Geometry check sheet. Reference: the model listing, model coordinates, mm. Face numbers are marked on the shaded views. A direction names the side the tool comes from. Give positions to 0.01 mm unless a question says otherwise; leave off trailing zeros. Order: outer loops, then holes, each group sorted by start corner. A loop starts at its lowest first (then second) coordinate and runs counter-clockwise, first axis right, second up.
from build123d import *

# Parameters (mm, degrees)
PAD_DEPTH       = 21
POCKET_DEPTH    = 5
POCKET001_DEPTH = 5
POCKET002_DEPTH = 10
SKETCH004_W     = 2.373045
SKETCH004_H     = 7.119136
POCKET003_DEPTH = 10
POCKET004_DEPTH = 10
POCKET005_DEPTH = 10
POCKET006_DEPTH = 2


with BuildPart() as part:
    # Sketch → Pad (new body)
    with BuildSketch(Plane.XY):
        Polygon((-10.032319, 15.304274), (9.936683, 15.304274), (19.912732, -0.173444), (9.919492, -15.052223), (9.919492, -25.320239), (-9.903072, -25.320239), (-9.903072, -15.596819), (-19.889567, -0.189549), align=None)
    extrude(amount=PAD_DEPTH)

    # Sketch001 (on Face10 of Pad) → Pocket (cut)
    with BuildSketch(Plane.XY.offset(21)):
        Polygon((-5.628046, 8.046473), (-9.278885, 3.056992), (-2.58568, 2.691908), align=None)
    extrude(amount=-POCKET_DEPTH, mode=Mode.SUBTRACT)

    # Sketch002 (on Face5 of Pocket) → Pocket001 (cut)
    with BuildSketch(Plane.XY.offset(21)):
        Polygon((6.8832, 8.120049), (3.658293, 3.373958), (10.594886, 3.069721), align=None)
    extrude(amount=-POCKET001_DEPTH, mode=Mode.SUBTRACT)

    # Sketch003 (on Face5 of Pocket001) → Pocket002 (cut)
    with BuildSketch(Plane.XY.offset(21)):
        Polygon((-7.814318, -23.860096), (-5.938107, -23.860096), (-5.938107, -16.355255), (-7.814318, -16.27368), align=None)
    extrude(amount=-POCKET002_DEPTH, mode=Mode.SUBTRACT)

    # Sketch004 (on Face5 of Pocket002) → Pocket003 (cut)
    with BuildSketch(Plane.XY.offset(21)):
        with Locations((-2.952688, -20.020277)):
            Rectangle(SKETCH004_W, SKETCH004_H)
    extrude(amount=-POCKET003_DEPTH, mode=Mode.SUBTRACT)

    # Sketch005 (on Face5 of Pocket003) → Pocket004 (cut)
    with BuildSketch(Plane.XY.offset(21)):
        Polygon((1.397894, -16.88661), (1.397894, -23.518969), (3.588397, -23.518969), (3.588397, -17.129999), align=None)
    extrude(amount=-POCKET004_DEPTH, mode=Mode.SUBTRACT)

    # Sketch006 (on Face5 of Pocket004) → Pocket005 (cut)
    with BuildSketch(Plane.XY.offset(21)):
        Polygon((5.109581, -16.88661), (5.474663, -23.701509), (7.847709, -23.823204), (7.847709, -16.460678), (5.474663, -16.704067), align=None)
    extrude(amount=-POCKET005_DEPTH, mode=Mode.SUBTRACT)

    # Sketch007 (on Face5 of Pocket005) → Pocket006 (cut)
    with BuildSketch(Plane.XY.offset(21)):
        Polygon((0, -2.312892), (-2.612413, -6.846357), (3.296795, -6.937919), align=None)
    extrude(amount=-POCKET006_DEPTH, mode=Mode.SUBTRACT)


solid = part.part
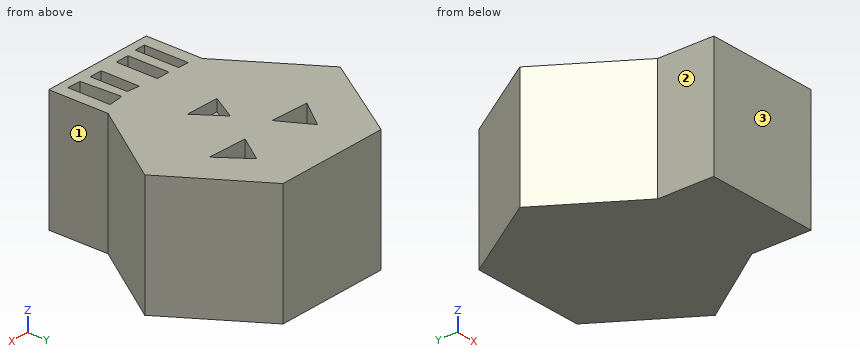
Item 1: Sectioned sample at C-C (y = 6.5). Enter the section's corners in (x, z), and give its area (3 significant figures).
Reported:
outline: (-15.63, 0) - (15.61, 0) - (15.61, 21) - (8.07, 21) - (8.07, 16) - (5.78, 16) - (5.78, 21) - (-4.75, 21) - (-4.75, 16) - (-6.76, 16) - (-6.76, 21) - (-15.63, 21) - close
area: 635 mm2
Item 2: Set-up check for the marked faces 1, 2 and 3: record each of +Z, -Z, +X, -X, +Y, -Y from which the full face is reachable in a straight line by a thin tool's end or side.
Reported:
face 1: +Z, -Z, +X, -Y
face 2: +Z, -Z, -X, -Y
face 3: +Z, -Z, +X, -X, -Y
Item 3: Scan lines: L1, parallel to X at y = 4, z = 19.75; L2, parallel to Y at x = 3.5, z = 14.5; L3, parallel to X at y = -21.5, z = 9.75. Record each from-to range of solid material in increasing order.
Reported:
L1: x = -17.22 to -8.59, -3.33 to 4.08, 9.91 to 17.22
L2: y = -25.32 to -23.52, -17.12 to 15.3
L3: x = -9.9 to 9.92
Item 4: Sectioned sample at A-A (z = 12.75). Enter the section's corners in (x, y), and give its area (3 significant figures).
Reported:
outline: (-19.89, -0.19) - (-9.9, -15.6) - (-9.9, -25.32) - (9.92, -25.32) - (9.92, -15.05) - (19.91, -0.17) - (9.94, 15.3) - (-10.03, 15.3) - close; hole (-7.81, -23.86) - (-5.94, -23.86) - (-5.94, -16.36) - (-7.81, -16.27) - close; hole (-4.14, -23.58) - (-1.77, -23.58) - (-1.77, -16.46) - (-4.14, -16.46) - close; hole (1.4, -23.52) - (3.59, -23.52) - (3.59, -17.13) - (1.4, -16.89) - close; hole (5.11, -16.89) - (5.47, -23.7) - (7.85, -23.82) - (7.85, -16.46) - (5.47, -16.7) - close
area: 1,050 mm2
Item 5: Gauge pin test, flat ends, axial feed: pin 1 (12 mm diameter, centred on x = -4.5, y = -11.5, fed in from -Z); pin 2 (10.5 mm diameter, centred on y = -22, z = 5.5, fed in from -X); pin 3 (6 mm diameter, centred on y = -19.5, z = 14.5, fed in from +X); pin 4 (2 mm diameter, centred on y = 2, z = 17, fed in from -X). Record the tip position at first contact, or that the pin passes through.
Reported:
pin 1: stops at z = 0
pin 2: stops at x = -9.9
pin 3: stops at x = 9.92
pin 4: stops at x = -19.13
Item 6: Sectioned sample at D-D (x = 17). Enter the section's corners in (y, z).
Reported:
outline: (-4.51, 0) - (4.35, 0) - (4.35, 21) - (-4.51, 21) - close
Item 7: Sectioned sample at B-B (z = 2). Enter the section's corners in (x, y).
Reported:
outline: (-19.89, -0.19) - (-9.9, -15.6) - (-9.9, -25.32) - (9.92, -25.32) - (9.92, -15.05) - (19.91, -0.17) - (9.94, 15.3) - (-10.03, 15.3) - close
